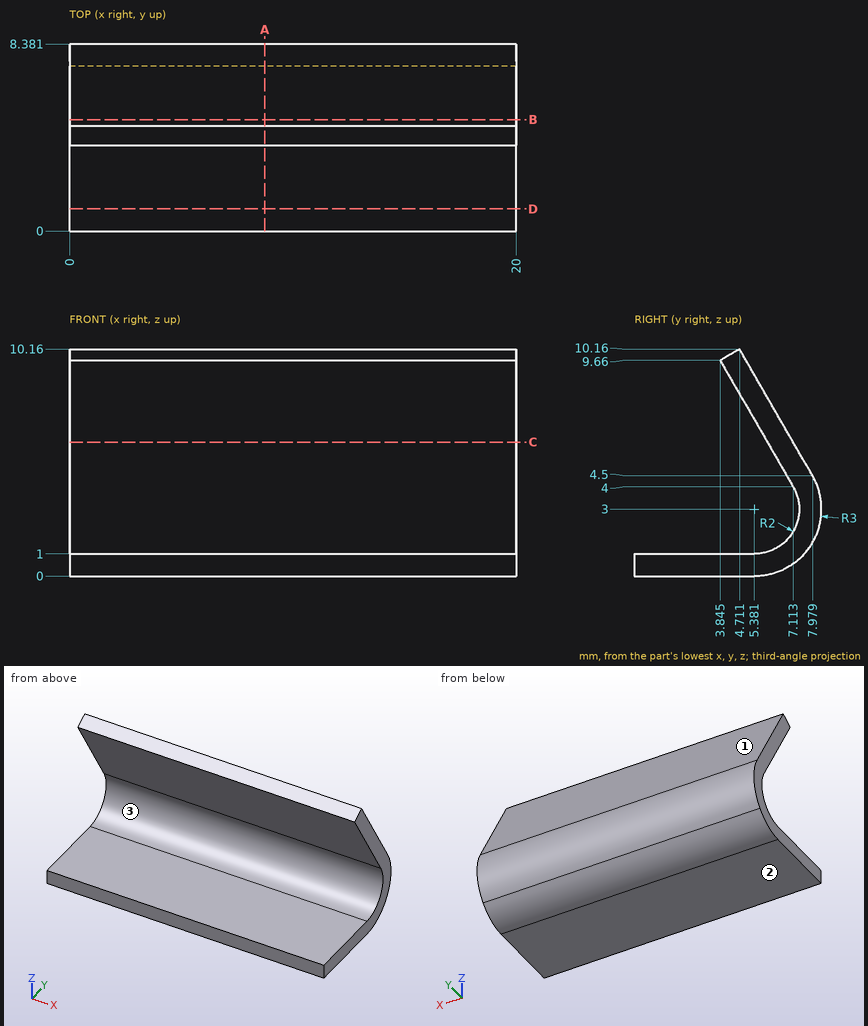
Can you work these out from the drawing? Everything is in mm from the part's minimum corner. Coordinates: 2 decimals unless noted, no trailing zeros. Order: outer loops, then holes, each group sorted by start corner. A loop starts at its lowest first (then second) coordinate and runs counter-clockwise, first axis right, second up. Notation, with made-up numbers: M 75,-12 L 90,-12 A19 cw 90,21 Z; hole C 16.5,66 d4. An arc over 180 degrees is marked long. Answer as CSV lines item,"result". Start each with the question number.
1. I want a section at B-B, the plane y = 5. Write out the boundary of the cut face in (x, z).
2. For pin 1 (4 mm diameter, centred on x = 15, z = 6.5, fed in from -Y) (1 decimal); pin 2 (5 mm diameter, centred on x = 18, z = 2.5, fed in from +Y); pin 3 (2.5 mm diameter, centred on x = 7.5, y = 3, fed in from +Z); pin 4 (1.5 mm diameter, centred on x = 5, z = 5.5, fed in from -Y) (1 decimal), each with a flat end and sliding along its axis, tell me the tip position at first contact or that it passes through.
3. I want a section at D-D, the plane y = 1. Write out the boundary of the cut face in (x, z).
4. I want a section at A-A, the plane x = 8.75. Write out the boundary of the cut face in (y, z) (1 decimal).
5. I need wall thicknesses on line 1 (Z direction, x = 10.75, y = 2.5); line 2 (Z direction, x = 7.75, y = 5); line 3 (Z direction, x = 11.25, y = 6.5) (1 decimal). Which ranges of each line are inside material? Lowest first, please. Write a range as [from, to].
6. I want a section at C-C, the plane z = 6. Write out the boundary of the cut face in (x, y), and give its area (3 significant figures).
7. We'd pull the mould along Z, two halves only. Please class the marked faces 1, 2 and 3: released by +Z, released by -Z, zero draft, split by the parting line, or undercut.
Recorded:
1,outline,"M 0,0 L 20,0 L 20,1 L 0,1 Z; M 0,7.66 L 20,7.66 L 20,9.66 L 0,9.66 Z"
2,pin 1,"stops at y = 4.5"
2,pin 2,"stops at y = 8.38"
2,pin 3,"stops at z = 9.89"
2,pin 4,"stops at y = 5.8"
3,outline,"M 0,0 L 20,0 L 20,1 L 0,1 Z"
4,outline,"M 0,0 L 5.4,0 A3 ccw 8,4.5 L 4.7,10.2 L 3.8,9.7 L 7.1,4 A2 cw 5.4,1 L 0,1 Z"
5,line 1,"z = [0, 1]"
5,line 2,"z = [0, 1], [7.66, 9.66]"
5,line 3,"z = [0.2, 1.3], [5.1, 7.1]"
6,outline,"M 0,5.96 L 20,5.96 L 20,7.11 L 0,7.11 Z"
6,area,"23.1 mm2"
7,face 1,"released by +Z"
7,face 2,"released by -Z"
7,face 3,"undercut"
